```python
from build123d import *

# Parameters (mm, degrees)
SKETCH1_W           = 99
SKETCH1_H           = 46
SKETCH1_W_2         = 89
SKETCH1_H_2         = 44
BOSS_EXTRUDE1_DEPTH = 10
SKETCH2_W           = 99
SKETCH2_H           = 1.5
BOSS_EXTRUDE2_DEPTH = 1.5
SKETCH4_W           = 6
SKETCH4_H           = 44
BOSS_EXTRUDE3_DEPTH = 4
SKETCH5_R           = 1.5
CUT_EXTRUDE1_DEPTH  = 4
SKETCH6_W           = 6
SKETCH6_H           = 44
CUT_EXTRUDE2_DEPTH  = 1
CUT_EXTRUDE3_REACH  = 104.476
SKETCH7_W           = 14
SKETCH7_H           = 3
SWEEP3_PROFILE_R    = 1.5
SKETCH23_R          = 1.5
CUT_EXTRUDE4_DEPTH  = 10


with BuildPart() as part:
    # Sketch1 → Boss-Extrude1 (new body)
    with BuildSketch(Plane(origin=(0, 0, 0), x_dir=(1, 0, 0), z_dir=(0, 1, 0))):
        Rectangle(SKETCH1_W, SKETCH1_H)
        Rectangle(SKETCH1_W_2, SKETCH1_H_2, mode=Mode.SUBTRACT)
    extrude(amount=BOSS_EXTRUDE1_DEPTH)

    # Sketch2 → Boss-Extrude2 (add)
    with BuildSketch(Plane.XY.offset(23)):
        with Locations((0, 2.75)):
            Rectangle(SKETCH2_W, SKETCH2_H)
        with Locations((0, 7.25)):
            Rectangle(SKETCH2_W, SKETCH2_H)
    boss_extrude2 = extrude(amount=BOSS_EXTRUDE2_DEPTH)

    # Mirror1: Boss-Extrude2 across plane
    add(boss_extrude2.mirror(Plane.XY))

    # Sketch4 → Boss-Extrude3 (add)
    with BuildSketch(Plane(origin=(0, 0, 0), x_dir=(1, 0, 0), z_dir=(0, 1, 0))):
        with Locations((-41.5, 0)):
            Rectangle(SKETCH4_W, SKETCH4_H)
    boss_extrude3 = extrude(amount=BOSS_EXTRUDE3_DEPTH)

    # Mirror2: Boss-Extrude3 across plane
    add(boss_extrude3.mirror(Plane(origin=(0, 0, 0), x_dir=(0, 0, 1), z_dir=(1, 0, 0))))

    # Sketch5 → Cut-Extrude1 (cut)
    with BuildSketch(Plane(origin=(0, 4, 0), x_dir=(1, 0, 0), z_dir=(0, 1, 0))):
        with Locations(Location((-41.75, 18.75, 0), (0, 0, 270))):
            Circle(SKETCH5_R)
        with Locations(Location((-41.75, -18.75, 0), (0, 0, 90))):
            Circle(SKETCH5_R)
    cut_extrude1 = extrude(amount=-CUT_EXTRUDE1_DEPTH, mode=Mode.SUBTRACT)

    # Mirror3: Cut-Extrude1 across plane
    add(cut_extrude1.mirror(Plane(origin=(0, 0, 0), x_dir=(0, 0, 1), z_dir=(1, 0, 0))), mode=Mode.SUBTRACT)

    # Sketch6 → Cut-Extrude2 (cut)
    with BuildSketch(Plane.XZ):
        with Locations((-41.5, 0)):
            Rectangle(SKETCH6_W, SKETCH6_H)
        with Locations((41.5, 0)):
            Rectangle(SKETCH6_W, SKETCH6_H)
    extrude(amount=-CUT_EXTRUDE2_DEPTH, mode=Mode.SUBTRACT)

    # Cut-Extrude3: up to this face of the body (flat: up to its plane)
    cut_extrude3_end = Plane(part.part.faces().sort_by_distance((38.5, 2.5, 0))[0])
    # Sketch7 → Cut-Extrude3 (cut, up to the picked face)
    with BuildSketch(Plane(origin=(49.5, 0, 0), x_dir=(0, 0, -1), z_dir=(1, 0, 0)), mode=Mode.PRIVATE) as cut_extrude3_sk1:
        with Locations((0, 1.5)):
            Rectangle(SKETCH7_W, SKETCH7_H)
    cut_extrude3_tool1 = split(extrude(cut_extrude3_sk1.sketch, amount=-CUT_EXTRUDE3_REACH, mode=Mode.PRIVATE), bisect_by=cut_extrude3_end, keep=Keep.BOTH, mode=Mode.PRIVATE)
    add(cut_extrude3_tool1.solids().sort_by(Axis((49.5, 1.5, 0), (-1, 0, 0)))[0], mode=Mode.SUBTRACT)

    # Sweep3: sweep along a path in Sketch9
    with BuildLine(Plane(origin=(0, 6, 0), x_dir=(1, 0, 0), z_dir=(0, 1, 0))) as sweep3_path:
        Line((49.5, 12.5), (52.5, 12.5))
        ThreePointArc((52.5, 12.5), (54.621320344, 11.621320344), (55.5, 9.5))
        Line((55.5, 9.5), (55.5, -9.5))
        ThreePointArc((55.5, -9.5), (54.621320344, -11.621320344), (52.5, -12.5))
        Line((52.5, -12.5), (49.5, -12.5))
    # Sweep3 profile (on start of the path) → Sweep3 (sweep)
    with BuildSketch(Plane(origin=(49.5, 6, -12.5), x_dir=(0, 0, 1), z_dir=(1, 0, 0))):
        Circle(SWEEP3_PROFILE_R)
    sweep(path=sweep3_path.line)

    # Sketch23 → Cut-Extrude4 (cut)
    with BuildSketch(Plane(origin=(0, 10, 0), x_dir=(1, 0, 0), z_dir=(0, 1, 0))):
        with Locations(Location((47, 18, 0), (0, 0, 270))):
            Circle(SKETCH23_R)
    extrude(amount=-CUT_EXTRUDE4_DEPTH, mode=Mode.SUBTRACT)


solid = part.part
```
Input: part model. Units: mm. Frame: model coordinates. A direction names the side the tool comes from. Give positions to 0.01 mm unless a question says otherwise; leave off trailing zeros. Loops run counter-clockwise (first coordinate to the right, second up) from the corner with the lowest first, then second, coordinate; pieces in that order, holes last. Notation, with made-up numbers: (49, 80) -> (58, 80) arc R29 ccw to (58, 102) -> close; hole circle Ø9 at (68.5, 32). An arc over 180 degrees is marked (long way). Use a Markdown table: item, result.
Q1. Section query A-A, the plane x = 47. Return the cut outline in (y, z), plus the area to 3 significant figures.
Entries:
| item | result |
|---|---|
| outline | (0, -23) -> (2, -23) -> (2, -24.5) -> (3.5, -24.5) -> (3.5, -23) -> (6.5, -23) -> (6.5, -24.5) -> (8, -24.5) -> (8, -23) -> (10, -23) -> (10, -19.5) -> (0, -19.5) -> close; (0, -16.5) -> (10, -16.5) -> (10, 23) -> (8, 23) -> (8, 24.5) -> (6.5, 24.5) -> (6.5, 23) -> (3.5, 23) -> (3.5, 24.5) -> (2, 24.5) -> (2, 23) -> (0, 23) -> (0, 7) -> (3, 7) -> (3, -7) -> (0, -7) -> close |
| area | 397 mm² |
Q2. Pull-direction query (Z, two-part tool) for faces 1 (the flat face through (42, 4, 0)), 2 (the flat face through (-0.2, 10, -22.3)), 3 (the flat face through (-1, 1, 23)); classes: pulls with the +Z half, pulls with the -Z half, needs draft (parallel to the pull), parting line crosses it, or undercut.
Entries:
| item | result |
|---|---|
| face 1 | undercut |
| face 2 | needs draft |
| face 3 | pulls with the +Z half |
Q3. First-contact query: P1, Ø2, axis at x = -11.5, y = 9.5, coming from the -Z side; P2, Ø1.8, axis at x = -41.5, z = -4, coming from the +Y side; P3, Ø2.5, axis at y = 2, z = -10.5, coming from the +X side; P4, Ø8, axis at x = -31, z = 13.5, coming from the +Y side. Flat tips, straight axial feed; report the tip coordinate or a pass-through.
Entries:
| item | result |
|---|---|
| P1 | stops at z = -23 |
| P2 | stops at y = 4 |
| P3 | stops at x = 49.5 |
| P4 | passes through |
Q4. Section query D-D, the plane x = -1. Return the cut outline in (y, z).
Entries:
| item | result |
|---|---|
| outline | (0, -23) -> (2, -23) -> (2, -24.5) -> (3.5, -24.5) -> (3.5, -23) -> (6.5, -23) -> (6.5, -24.5) -> (8, -24.5) -> (8, -23) -> (10, -23) -> (10, -22) -> (0, -22) -> close; (0, 22) -> (10, 22) -> (10, 23) -> (8, 23) -> (8, 24.5) -> (6.5, 24.5) -> (6.5, 23) -> (3.5, 23) -> (3.5, 24.5) -> (2, 24.5) -> (2, 23) -> (0, 23) -> close |
Q5. Section query C-C, the plane z = 1. Return the cut outline in (x, y).
Entries:
| item | result |
|---|---|
| outline | (-49.5, 0) -> (-44.5, 0) -> (-44.5, 1) -> (-38.5, 1) -> (-38.5, 4) -> (-44.5, 4) -> (-44.5, 10) -> (-49.5, 10) -> close; (38.5, 3) -> (49.5, 3) -> (49.5, 10) -> (44.5, 10) -> (44.5, 4) -> (38.5, 4) -> close; circle Ø3 at (55.5, 6) |
Q6. Section query B-B, the plane z = 18.75. Return the cut outline in (x, y), plus the area to 3 significant figures.
Entries:
| item | result |
|---|---|
| outline | (-49.5, 0) -> (-44.5, 0) -> (-44.5, 1) -> (-43.25, 1) -> (-43.25, 4) -> (-44.5, 4) -> (-44.5, 10) -> (-49.5, 10) -> close; (-40.25, 1) -> (-38.5, 1) -> (-38.5, 4) -> (-40.25, 4) -> close; (38.5, 1) -> (40.25, 1) -> (40.25, 4) -> (38.5, 4) -> close; (43.25, 1) -> (44.5, 1) -> (44.5, 0) -> (49.5, 0) -> (49.5, 10) -> (44.5, 10) -> (44.5, 4) -> (43.25, 4) -> close |
| area | 118 mm² |
Q7. Access query for faces 4 (the flat face through (-42, 1, 0)), 5 (the flat face through (38.5, 3.5, 0.3)), 6 (the flat face through (-1, 9, -23)). Directions: +Z, -Z, +X, -X, +Y, -Y. A direction counts if a zero-diameter tool reaches every point of the face in a straight line with its end or side. Return the directions, or none.
Entries:
| item | result |
|---|---|
| face 4 | -Y |
| face 5 | +Y, -Y |
| face 6 | -Z, +X, -X, +Y |
Q8. Ray query, probe 1 along Z at (x, y) = (41.75, 2.55); probe 2 along X at (y, z) = (7.75, -18); probe 3 along X at (y, z) = (5.75, -9). Return the intervals inside material, ascending. Write a range as from..to.
Entries:
| item | result |
|---|---|
| probe 1 | z = -24.5..-20.25, -17.25..-7, 7..17.25, 20.25..24.5 |
| probe 2 | x = -49.5..-44.5, 44.5..45.5, 48.5..49.5 |
| probe 3 | x = -49.5..-44.5, 44.5..49.5, 54.02..56.98 |
